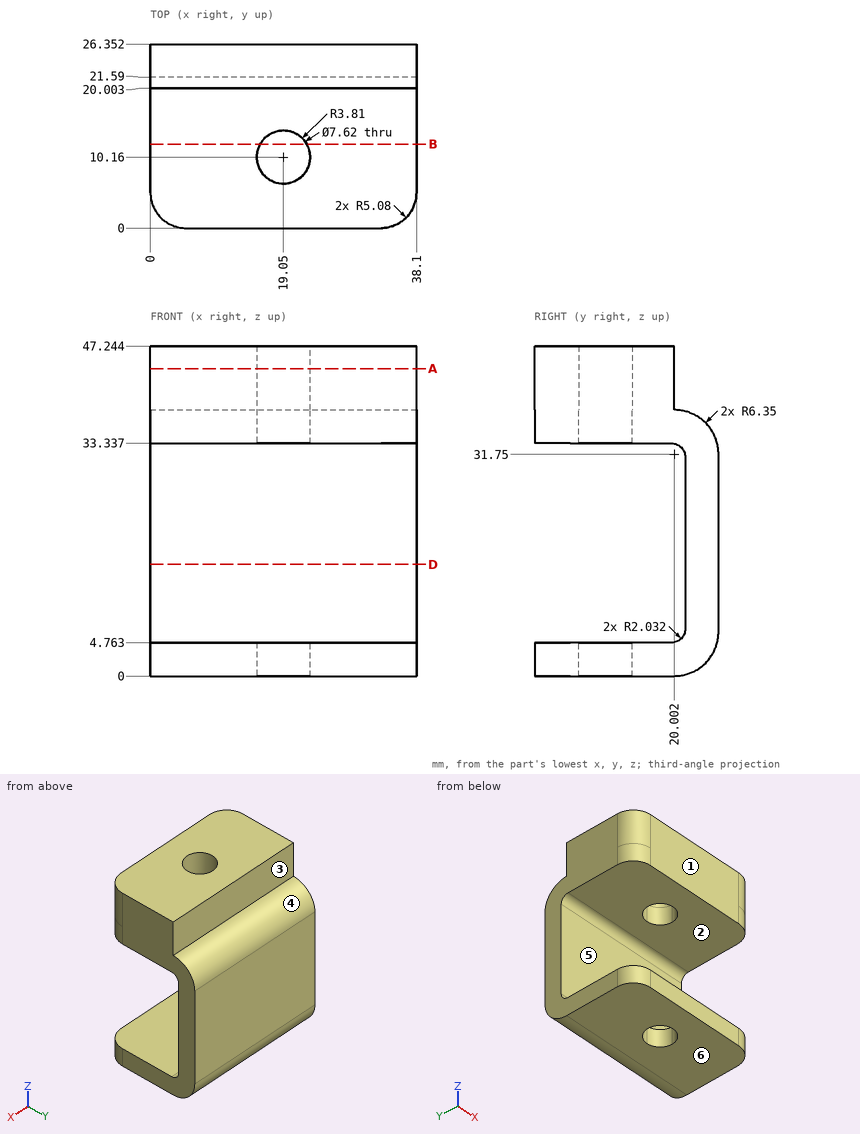
The drawing under review shows one solid part. Ordinate dimensions are in mm from its lowest x, y, z. A direction names the side the tool comes from. Round coordinates to 2 decimals unless told otherwise and drop trailing zeros. Write each loop counter-clockwise with the first axis right and the second up, starting at its lowest first coordinate (ties: lowest second). Pieces come first, ordered by that corner, then holes.
(1) We need section D-D on z = 16. Give the boundary of the cut face in (x, y).
(2) Wall thickness on L1, parallel to Z at x = 34, y = 16 (1 decimal); L2, parallel to X at y = 10.16, z = 41.5; L3, parallel to Y at x = 19.05, z = 42.5: over which ranges is each line inside the solid? List them lowest first.
(3) Machinability: for the marked faces 1 and 2, which of the approach directions +Z, -Z, +X, -X, +Y, -Y give a long, thin tool a straight path to every point of the face, cutting with its end or side? Answer none if there is none.
(4) We need section B-B on y = 12. Give the boundary of the cut face in (x, z) (1 decimal).
(5) Mouldability with a two-part tool opening along Z and no side actions: class the marked faces 3, 4, 5 and 6 as +Z half, -Z half, draft (parallel to the pull), parting line (faces both ways), or undercut.
(6) Insertion check: pin 1 (10 mm diameter, centred on x = 17, z = 41.5, fed in from +Y) (1 decimal); pin 2 (6 mm diameter, centred on x = 19.05, y = 10.16, fed in from -Z); pin 3 (12 mm diameter, centred on x = 9, z = 38, fed in from +Y). Each pin has a flat end and moves straight along its axis. Give the tip position at first contact, or say it passes through.
(7) We need section A-A on z = 44. Give the boundary of the cut face in (x, y).
Findings below:
1. outline: (0, 21.59) - (38.1, 21.59) - (38.1, 26.35) - (0, 26.35) - close
2. L1: z = 0 to 4.8, 33.3 to 47.2
2. L2: x = 0 to 15.24, 22.86 to 38.1
2. L3: y = 0 to 6.35, 13.97 to 20
3. face 1: +Z, -Z, +X, -X, -Y
3. face 2: +X, -X, -Y
4. outline: (0, 0) - (15.7, 0) - (15.7, 4.8) - (0, 4.8) - close; (0, 33.3) - (15.7, 33.3) - (15.7, 47.2) - (0, 47.2) - close; (22.4, 0) - (38.1, 0) - (38.1, 4.8) - (22.4, 4.8) - close; (22.4, 33.3) - (38.1, 33.3) - (38.1, 47.2) - (22.4, 47.2) - close
5. face 3: draft
5. face 4: +Z half
5. face 5: undercut
5. face 6: -Z half
6. pin 1: stops at y = 24.2
6. pin 2: passes through
6. pin 3: stops at y = 26.35
7. outline: (0, 5.08) arc R5.08 ccw to (5.08, 0) - (33.02, 0) arc R5.08 ccw to (38.1, 5.08) - (38.1, 20) - (0, 20) - close; hole circle Ø7.62 at (19.05, 10.16)
